Print and shaded views of the part. All mm, measured from the part's lowest x, y and z. Round coordinates to 2 decimals unless told otherwise and drop trailing zeros. Order: outer loops, then holes, each group sorted by start corner. A loop starts at its lowest first (then second) coordinate and runs counter-clockwise, first axis right, second up. Notation, with made-up numbers: (7, -8.75) - (40, -8.75) arc R11 cw to (40, -0.75) - close; hole circle Ø9 at (-18.5, 59.25). An arc over 180 degrees is marked (long way). Write item = value, one per line.
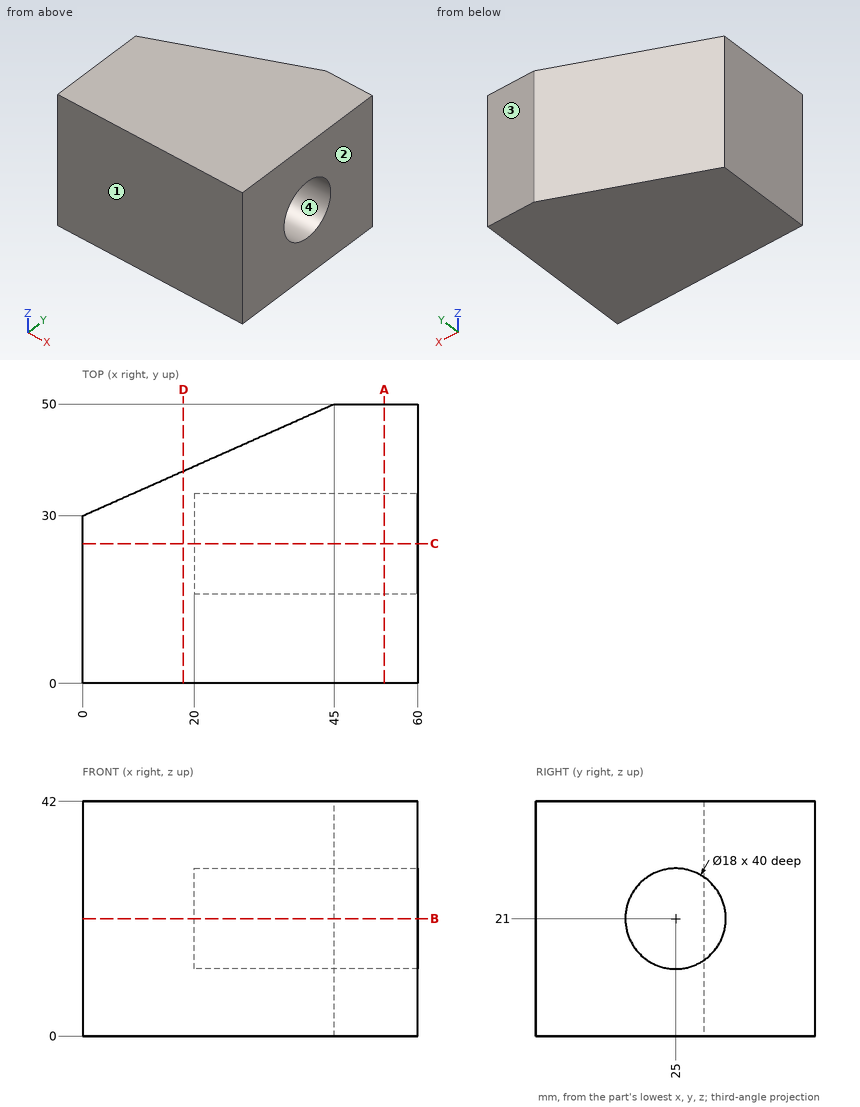
(1) Probe line 1 along Y through (x, z) = (36.5, 21); line 2 along Z through (x, y) = (48, 22.5); line 3 along Y through (x, z) = (37, 21). List the from-to ranges inside material, lowest first.
Solved:
line_1 = 0 to 16, 34 to 46.22
line_2 = 0 to 12.35, 29.65 to 42
line_3 = 0 to 16, 34 to 46.44
(2) Band-saw the part on D-D on x = 18. List the corners of the cut face in (y, z).
Solved:
outline = (0, 0) - (38, 0) - (38, 42) - (0, 42) - close
(3) Band-saw the part on C-C on y = 25. List the corners of the cut face in (x, z).
Solved:
outline = (0, 0) - (60, 0) - (60, 12) - (20, 12) - (20, 30) - (60, 30) - (60, 42) - (0, 42) - close
(4) Band-saw the part on A-A on x = 54. List the corners of the cut face in (y, z), plus the area to 3 significant figures.
Solved:
outline = (0, 0) - (50, 0) - (50, 42) - (0, 42) - close; hole circle Ø18 at (25, 21)
area = 1,850 mm²
(5) Pull direction Y, two halves, no side cores. Call the marked faces 1, 2, 3 and 4: released by +Y, released by -Y, zero draft, split by the parting line, or undercut.
Solved:
face_1 = released by -Y
face_2 = zero draft
face_3 = released by +Y
face_4 = undercut
(6) Band-saw the part on B-B on z = 21. List the corners of the cut face in (x, y).
Solved:
outline = (0, 0) - (60, 0) - (60, 16) - (20, 16) - (20, 34) - (60, 34) - (60, 50) - (45, 50) - (0, 30) - close
(7) Drop a flat-ended pin along its axis: pin 1 (3 mm diameter, centred on x = 20.5, z = 25, fed in from +Y). Give the stop position or say it passes through.
Solved:
pin_1 = 39.78
